Work out the finished part from the listing and answer in its coordinate system (mm). Face numbers are marked on the shaded views. A direction names the side the tool comes from. Coordinates: 2 decimals unless noted, no trailing zeros. Write each loop counter-clockwise with the first axis right and the second up, starting at its lowest first coordinate (ties: lowest second). Pieces come first, ordered by that corner, then holes. Notation, with made-up numbers: (2.5, -25) -> (34.5, -25) arc R17 cw to (34.5, 1) -> close; hole circle Ø1 at (79, 32). An arc over 180 degrees is marked (long way). Write each question's results on one line, items separated by ' | '. Start each with the question number.
from build123d import *

# Parameters (mm, degrees)
EXTRUDE_2_DEPTH              = 67
CUT_EXTRUDE_5_DEPTH          = 15
CUT_EXTRUDE_6_DEPTH          = 15
SKETCH_4_W                   = 15
SKETCH_4_H                   = 47
CUT_EXTRUDE_7_DEPTH          = 100
CUT_EXTRUDE_8_DEPTH          = 100
CUT_EXTRUDE_11_DEPTH         = 25
CUT_EXTRUDE_12_DEPTH         = 25
CUT_EXTRUDE_13_DEPTH         = 25
CUT_EXTRUDE_14_DEPTH         = 25
HOLE_WIZARD_M5_1_D           = 5.5
HOLE_WIZARD_M5_1_CBORE_D     = 9.5
HOLE_WIZARD_M5_1_CBORE_DEPTH = 5
SKETCH_24_R                  = 1.25
CUT_EXTRUDE_15_DEPTH         = 50
SKETCH_25_W                  = 20
SKETCH_25_H                  = 10
CUT_EXTRUDE_16_DEPTH         = 100


with BuildPart() as part:
    # 스케치1 → 보스-돌출2 (new body)
    with BuildSketch(Plane.XY):
        with BuildLine():
            Line((0, 85.5), (0, 52.75))
            Line((0, 52.75), (-52.75, 0))
            Line((-52.75, 0), (-135.5, 0))
            Line((-135.5, 0), (-135.5, -15))
            Line((-135.5, -15), (-115.5, -15))
            Line((-115.5, -15), (-115.5, -25))
            Line((-115.5, -25), (-85.5, -25))
            Line((-85.5, -25), (-85.5, -15))
            Line((-85.5, -15), (-10, -15))
            Line((-10, -15), (-10, -25))
            Line((-10, -25), (0, -25))
            Line((0, -25), (0, -15))
            Line((0, -15), (15, 0))
            Line((15, 0), (25, 0))
            Line((25, 0), (25, 10))
            ThreePointArc((25, 10), (14.393398282, 14.393398282), (10, 25))
            Line((10, 25), (10, 60.5))
            ThreePointArc((10, 60.5), (14.393398282, 71.106601718), (25, 75.5))
            Line((25, 75.5), (25, 85.5))
            Line((25, 85.5), (0, 85.5))
        make_face()
        Polygon((-42.75, 0), (0, 42.75), (0, 0), align=None, mode=Mode.SUBTRACT)
    extrude(amount=EXTRUDE_2_DEPTH)

    # 스케치2 → 컷-돌출5 (cut)
    with BuildSketch(Plane.XY.offset(67)):
        Polygon((0, 52.75), (0, 42.75), (-42.75, 0), (-52.75, 0), align=None)
    extrude(amount=-CUT_EXTRUDE_5_DEPTH, mode=Mode.SUBTRACT)

    # 스케치3 → 컷-돌출6 (cut)
    with BuildSketch(Plane(origin=(0, 0, 0), x_dir=(-1, 0, 0), z_dir=(0, 0, -1))):
        Polygon((0, 52.75), (0, 42.75), (42.75, 0), (52.75, 0), align=None)
    extrude(amount=-CUT_EXTRUDE_6_DEPTH, mode=Mode.SUBTRACT)

    # 스케치4 → 컷-돌출7 (cut)
    with BuildSketch(Plane(origin=(0, 85.5, 0), x_dir=(1, 0, 0), z_dir=(0, 1, 0))):
        with Locations((17.5, -33.5)):
            Rectangle(SKETCH_4_W, SKETCH_4_H)
    extrude(amount=-CUT_EXTRUDE_7_DEPTH, mode=Mode.SUBTRACT)

    # 스케치5 → 컷-돌출8 (cut)
    with BuildSketch(Plane(origin=(0, 0, 0), x_dir=(1, 0, 0), z_dir=(0, 1, 0))):
        with BuildLine():
            ThreePointArc((-135.5, -34), (-135, -33.5), (-135.5, -33))
            Line((-135.5, -33), (-135.5, -33.5))
            Line((-135.5, -33.5), (-135.5, -34))
        make_face()
    extrude(amount=-CUT_EXTRUDE_8_DEPTH, mode=Mode.SUBTRACT)

    # 스케치8 → 컷-돌출11 (cut)
    with BuildSketch(Plane(origin=(25, 0, 0), x_dir=(0, 0, -1), z_dir=(1, 0, 0))):
        with BuildLine():
            ThreePointArc((-60, 80.5), (-62, 82.5), (-64, 80.5))
            Line((-64, 80.5), (-60, 80.5))
        make_face()
        with BuildLine():
            Line((-60, 80.5), (-64, 80.5))
            ThreePointArc((-64, 80.5), (-62, 78.5), (-60, 80.5))
        make_face()
    extrude(amount=-CUT_EXTRUDE_11_DEPTH, mode=Mode.SUBTRACT)

    # 스케치10 → 컷-돌출12 (cut)
    with BuildSketch(Plane(origin=(25, 0, 0), x_dir=(0, 0, -1), z_dir=(1, 0, 0))):
        with BuildLine():
            ThreePointArc((-3, 80.5), (-5, 82.5), (-7, 80.5))
            Line((-7, 80.5), (-3, 80.5))
        make_face()
        with BuildLine():
            Line((-3, 80.5), (-7, 80.5))
            ThreePointArc((-7, 80.5), (-5, 78.5), (-3, 80.5))
        make_face()
    extrude(amount=-CUT_EXTRUDE_12_DEPTH, mode=Mode.SUBTRACT)

    # 스케치11 → 컷-돌출13 (cut)
    with BuildSketch(Plane(origin=(25, 0, 0), x_dir=(0, 0, -1), z_dir=(1, 0, 0))):
        with BuildLine():
            ThreePointArc((-64, 5), (-62, 3), (-60, 5))
            Line((-60, 5), (-64, 5))
        make_face()
        with BuildLine():
            Line((-64, 5), (-60, 5))
            ThreePointArc((-60, 5), (-62, 7), (-64, 5))
        make_face()
    extrude(amount=-CUT_EXTRUDE_13_DEPTH, mode=Mode.SUBTRACT)

    # 스케치12 → 컷-돌출14 (cut)
    with BuildSketch(Plane(origin=(25, 0, 0), x_dir=(0, 0, -1), z_dir=(1, 0, 0))):
        with BuildLine():
            ThreePointArc((-7, 5), (-5, 3), (-3, 5))
            Line((-3, 5), (-7, 5))
        make_face()
        with BuildLine():
            Line((-7, 5), (-3, 5))
            ThreePointArc((-3, 5), (-5, 7), (-7, 5))
        make_face()
    extrude(amount=-CUT_EXTRUDE_14_DEPTH, mode=Mode.SUBTRACT)

    # M5 소켓 머리 캡 나사용 카운터보어1 (through all)
    with Locations(Plane(origin=(0, 0, 0), x_dir=(1, 0, 0), z_dir=(0, 1, 0))):
        with Locations((-125.5, -10), (-125.5, -57), (-20, -10), (-20, -57)):
            CounterBoreHole(HOLE_WIZARD_M5_1_D / 2, HOLE_WIZARD_M5_1_CBORE_D / 2, HOLE_WIZARD_M5_1_CBORE_DEPTH)

    # 스케치24 → 컷-돌출15 (cut)
    with BuildSketch(Plane(origin=(0, 0, 0), x_dir=(1, 0, 0), z_dir=(0, 1, 0))):
        with Locations(Location((-62.75, -33.5, 0), (0, 0, 180))):
            Circle(SKETCH_24_R)
        with Locations(Location((-92.75, -33.5, 0), (0, 0, 180))):
            Circle(SKETCH_24_R)
    extrude(amount=-CUT_EXTRUDE_15_DEPTH, mode=Mode.SUBTRACT)

    # 스케치25 → 컷-돌출16 (cut)
    with BuildSketch(Plane(origin=(0, 0, 0), x_dir=(-1, 0, 0), z_dir=(0, 0, -1))):
        with Locations((95.5, -20)):
            Rectangle(SKETCH_25_W, SKETCH_25_H)
    extrude(amount=-CUT_EXTRUDE_16_DEPTH, mode=Mode.SUBTRACT)


solid = part.part
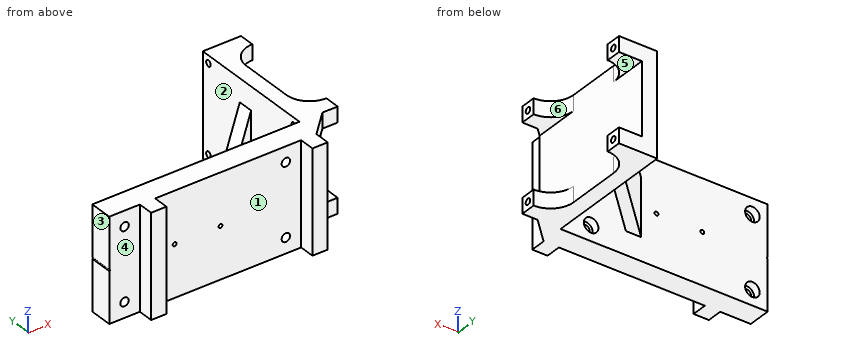
1. Determine the mould class of the marked faces 1, 2 and 3 for opening direction Y: pulls with the +Y half, pulls with the -Y half, needs draft (parallel to the pull), parting line crosses it, or undercut.
2. Find section A-A on y = 38. Give the vertices of the cut face in (x, z), and give its area (3 significant figures).
3. Find section D-D on x = -37.5. Give the vertices of the cut face in (y, z), and give its area (4 significant figures).
4. Given pin 1 Ø3 at (x, z) = (-124, 8.5) entering from +Y; pin 2 Ø8 at (x, y) = (-49.5, 10) entering from -Z; pin 3 Ø11 at (y, z) = (-19.5, 37.5) entering from +X; pin 4 Ø1.5 at (x, z) = (-68.5, 16) entering from -Y, each flat-ended and moving along its own axis, determine where each tip first touches the part or whether it passes through.
5. For the marked faces 4, 5 and 6, determine the directions among +Z, -Z, +X, -X, +Y, -Y from which every point of the face is accessible in a straight line to the end or side of a thin tool.
6. Find section B-B on x = -125.5. Give the vertices of the cut face in (y, z).
7. Find the intervals of material crossed by L1, parallel to Z at x = 13.5, y = 80.5; L2, parallel to X at y = -7.25, z = 10; L3, parallel to Y at x = 17, z = 62, in increasing order.
8. Find section C-C on y = 5. Give the vertices of the cut face in (x, z).
Ans:
1) face 1: pulls with the -Y half | face 2: undercut | face 3: needs draft
2) outline: (-14.75, 15) -> (-4.75, 15) -> (-4.75, 52) -> (-14.75, 52) -> close; (0, 0) -> (10, 0) -> (10, 67) -> (0, 67) -> close | area: 1,040 mm²
3) outline: (-15, 0) -> (0, 0) -> (0, 67) -> (-15, 67) -> close; (5.25, 15) -> (15.25, 15) -> (15.25, 52) -> (5.25, 52) -> close | area: 1,375 mm²
4) pin 1: stops at y = -5 | pin 2: passes through | pin 3: stops at x = 1 | pin 4: stops at y = -15
5) face 4: +Z, -Z, -X, -Y | face 5: +X, +Y, -Y | face 6: +Z, -Z, +X
6) outline: (-15, 0) -> (0, 0) -> (0, 5.25) -> (-5, 5.25) -> (-5, 7.25) -> (-15, 7.25) -> close; (-15, 12.75) -> (-5, 12.75) -> (-5, 14.75) -> (0, 14.75) -> (0, 52.25) -> (-5, 52.25) -> (-5, 54.25) -> (-15, 54.25) -> close; (-15, 59.75) -> (-5, 59.75) -> (-5, 61.75) -> (0, 61.75) -> (0, 67) -> (-15, 67) -> close
7) L1: z = 0 to 3, 7 to 10, 57 to 60, 64 to 67 | L2: x = -135.5 to -128.25, -122.75 to -22.75, -17.25 to 7.75 | L3: y = 0 to 3, 7 to 12.31, 73.19 to 78.5, 82.5 to 85.5
8) outline: (-47.75, 15) -> (-37.75, 15) -> (-37.75, 52) -> (-47.75, 52) -> close; (0, 0) -> (25, 0) -> (25, 3) -> (0, 3) -> close; (0, 7) -> (25, 7) -> (25, 10) -> (10, 10) -> (10, 57) -> (25, 57) -> (25, 60) -> (0, 60) -> close; (0, 64) -> (25, 64) -> (25, 67) -> (0, 67) -> close
